Input: part model. Units: mm. Frame: model coordinates. Face numbers are marked on the shaded views. A direction names the side the tool comes from. Coordinates: 2 decimals unless noted, no trailing zeros. Write each loop counter-clockwise with the first axis right and the second up, starting at its lowest first coordinate (ties: lowest second). Pieces come first, ordered by that corner, then holes. Notation, with made-up numbers: (-19, 34.25) - (19, 34.25) arc R25 ccw to (19, 52.25) - close; hole circle Ø10 at (-26.5, 30.5). An arc over 180 degrees is marked (long way). Use a Markdown table: item, result. Add a question column.
Q1. Section query C-C (y = 0). Give the number of separate pieces and of enclosed holes in the cut face, then the cut area to 3 significant figures.
Q2. Section query A-A (z = 31). Return the cut outline in (x, y).
Q3. Mould query, pull axis X, two halves, no side actions, for the marked faces 3, 4 and 5. Classes: released by +X, released by -X, zero draft, split by the parting line, or undercut.
Q4. Pin query (flat end, axial travel): P1, Ø6, axis at x = 35.5, y = -2, coming from the +Z side; P2, Ø0.9, axis at y = -4.25, z = 25.25, coming from the -X side. Return the tip coordinate at first contact, or that it passes through.
Q5. Section query D-D (x = 5). Return the cut outline in (y, z), then the cut area to 3 significant figures.
Q6. Material intervals for probe 1 along X at (y, z) = (-4.25, 9); probe 2 along X at (y, z) = (0, 0.35) (1 decimal); probe 3 along Z at (x, y) = (13, 0), sorted ascending. Write a range as from..to.
Q7. Section query B-B (z = 20). Return the cut outline in (x, y), then the cut area to 3 significant figures.
Q8. Set-up query: the marked faces 1 and 2. Return all of +Z, -Z, +X, -X, +Y, -Y with unobstructed straight access to the full face (end or side cutting, diameter ignored); none if empty.
Solid Edge part; units mm, degrees
sketch "Sketch1" plane through (0, 0, 0) normal (0, -1, 0) x (1, 0, 0)
  line L0 (0, 0) -> (43.15, 0)
  line L1 (43.15, 0) -> (43.15, 26.5)
  line L2 (41.65, 26.5) -> (43.15, 26.5)
  line L3 (41.65, 1.5) -> (41.65, 26.5)
  line L4 (1.5, 1.5) -> (41.65, 1.5)
  line L5 (1.5, 33.45) -> (1.5, 1.5)
  line L6 (1.5, 33.45) -> (0, 33.45)
  line L7 (0, 0) -> (0, 33.45)
  dimension "D1" = 43.15
extrude "Protrusion1" add sketch "Sketch1" along normal mid plane 16
hole "Hole_1" at (43.15, 0, 21) direction (-1, 0, 0) diameter 4.1 end through all
hole "Hole_2" at (0, 0, 11) direction (1, 0, 0) diameter 1.075 end up to next
hole "Hole1" at (0, 0, 31) direction (1, 0, 0) diameter 1.075 end up to next
sketch "Sketch2" plane through (0, 0, 16.725) normal (-1, 0, 0) x (0, -1, 0)
  circle A0 centre (0, 4.275) radius 4
extrude "Cutout1" cut sketch "Sketch2" against normal up to next
hole "Hole_4" at (0, -4.25, 25.25) direction (1, 0, 0) diameter 1.075 end up to next
hole "Hole2" at (0, -4.25, 16.75) direction (1, 0, 0) diameter 1.075 end up to next
hole "Hole3" at (0, 4.25, 16.75) direction (1, 0, 0) diameter 1.075 end up to next
hole "Hole4" at (0, 4.25, 25.25) direction (1, 0, 0) diameter 1.075 end up to next
chamfer "Chamfer_1" distance 3 angle 45 4 edges at (0.75, 8, 33.45) (0.75, -8, 33.45) (42.4, 8, 26.5) (42.4, -8, 26.5)
fillet "Round_1" radius 2.5 2 edges at (0, 0, 0) (43.15, 0, 0)
hole "Hole_8" at (9.575, 4, 0) direction (0, 0, 1) diameter 3.2 end up to next
hole "Hole5" at (9.575, -4, 0) direction (0, 0, 1) diameter 3.2 end up to next
hole "Hole6" at (17.575, -4, 0) direction (0, 0, 1) diameter 3.2 end up to next
hole "Hole7" at (17.575, 4, 0) direction (0, 0, 1) diameter 3.2 end up to next
hole "Hole8" at (25.575, 4, 0) direction (0, 0, 1) diameter 3.2 end up to next
hole "Hole9" at (25.575, -4, 0) direction (0, 0, 1) diameter 3.2 end up to next
hole "Hole10" at (33.575, -4, 0) direction (0, 0, 1) diameter 3.2 end up to next
hole "Hole11" at (33.575, 4, 0) direction (0, 0, 1) diameter 3.2 end up to next
hole "Hole_16" at (21.575, 0, 0) direction (0, 0, 1) diameter 8.1 end up to next
hole "Hole_17" at (21.575, 6, 0) direction (0, 0, 1) diameter 1.075 end up to next
hole "Hole12" at (21.575, -6, 0) direction (0, 0, 1) diameter 1.075 end up to next
hole "Hole13" at (15.575, 0, 0) direction (0, 0, 1) diameter 1.075 end up to next
hole "Hole14" at (27.575, 0, 0) direction (0, 0, 1) diameter 1.075 end up to next
hole "Hole15" at (31.575, 0, 0) direction (0, 0, 1) diameter 1.075 end up to next
hole "Hole16" at (11.575, 0, 0) direction (0, 0, 1) diameter 1.075 end up to next
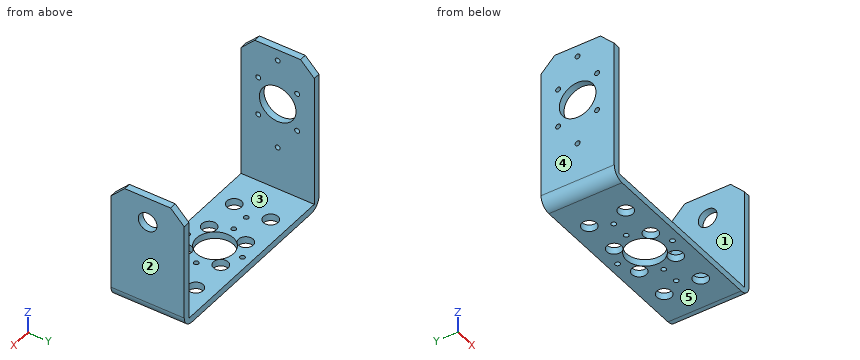
Values follow:
| question | item | result |
|---|---|---|
| 1 | separate pieces | 10 |
| 1 | enclosed holes | 0 |
| 1 | area | 107 mm2 |
| 2 | outline | (0, -7.45) - (1.5, -7.45) - (1.5, -0.54) - (0, -0.54) - close; (0, 0.54) - (1.5, 0.54) - (1.5, 7.45) - (0, 7.45) - close |
| 3 | face 3 | undercut |
| 3 | face 4 | released by -X |
| 3 | face 5 | zero draft |
| 4 | P1 | z = 1.5 |
| 4 | P2 | x = 41.65 |
| 5 | outline | (-8, 0) - (8, 0) - (8, 1.5) - (-8, 1.5) - close |
| 5 | area | 24.0 mm2 |
| 6 | probe 1 | 0..1.5, 41.65..43.15 |
| 6 | probe 2 | 1.2..11, 12.1..15, 16.1..17.5, 25.6..27, 28.1..31, 32.1..41.9 |
| 6 | probe 3 | 0..1.5 |
| 7 | outline | (0, -8) - (1.5, -8) - (1.5, -3.87) - (0, -3.87) - close; (0, 3.87) - (1.5, 3.87) - (1.5, 8) - (0, 8) - close; (41.65, -8) - (43.15, -8) - (43.15, -1.79) - (41.65, -1.79) - close; (41.65, 1.79) - (43.15, 1.79) - (43.15, 8) - (41.65, 8) - close |
| 7 | area | 31.0 mm2 |
| 8 | face 1 | +Z, +Y, -Y |
| 8 | face 2 | +Z, -Z, +X, +Y, -Y |
